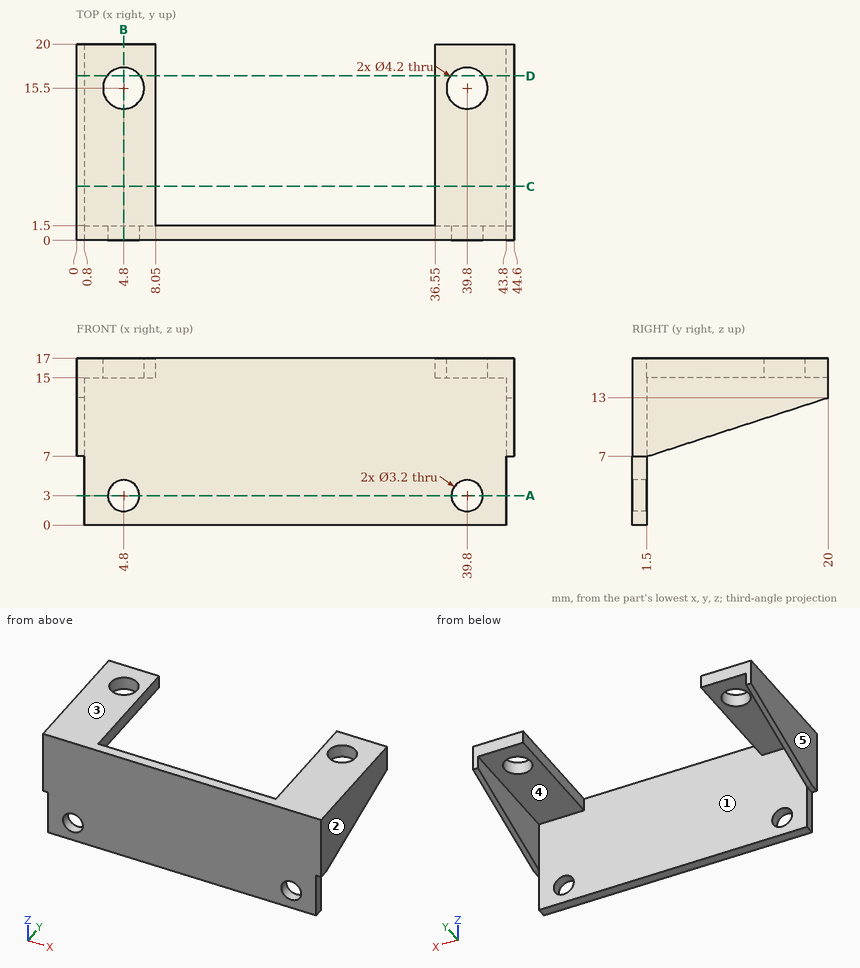
Input: dimensioned drawing with shaded views. Units: mm. Origin: part minimum x, y, z. A direction names the side the tool comes from. Coordinates: 2 decimals unless noted, no trailing zeros. Loops run counter-clockwise (first coordinate to the right, second up) from the corner with the lowest first, then second, coordinate; pieces in that order, holes last. Notation, with made-up numbers: M 83,-21.5 L 117,-21.5 A9 ccw 117,-13.5 Z; hole C 40.25,42 d8. An arc over 180 degrees is marked long. Use a Markdown table: item, result. Add a question column.
Q1. Section query D-D, the plane y = 16.75. Return loops of the section in (x, z).
Q2. Section query B-B, the plane x = 4.8. Return loops of the section in (y, z), and give its area (3 significant figures).
Q3. Material intervals for L1, parallel to X at y = 1, z = 3; L2, parallel to Y at x = 39.8, z = 16.1; L3, parallel to X at y = 3, z = 9.25, sorted ascending.
Q4. Draft query along X for the marked faces 1, 2 and 3. Return one class per face: pulls with the +X half, pulls with the -X half, needs draft (parallel to the pull), parting line crosses it, or undercut.
Q5. Access query for the marked faces 4 and 5. Directions: +Z, -Z, +X, -X, +Y, -Y. A direction counts if a zero-diameter tool reaches every point of the face in a straight line with its end or side. Return the directions, or none.
Q6. First-contact query: pin 1 (1.5 mm diameter, centred on x = 25, y = 3, fed in from +Z); pin 2 (0.8 mm diameter, centred on y = 1, z = 3, fed in from -X); pin 3 (12 mm diameter, centred on x = 13.5, y = 8, fed in from -Z); pin 4 (8 mm diameter, centred on x = 11.5, z = 4.5, fed in from +Y). Flat tips, straight axial feed; report the tip coordinate or a pass-through.
Q7. Section query C-C, the plane y = 5.5. Return loops of the section in (x, z).
Q8. Section query A-A, the plane z = 3. Return loops of the section in (x, y), and give its area (3 significant figures).
Result:
| question | item | result |
|---|---|---|
| 1 | outline | M 0,11.95 L 0.8,11.95 L 0.8,15 L 3.11,15 L 3.11,17 L 0,17 Z; M 6.49,15 L 8.05,15 L 8.05,17 L 6.49,17 Z; M 36.55,15 L 38.11,15 L 38.11,17 L 36.55,17 Z; M 41.49,15 L 43.8,15 L 43.8,11.95 L 44.6,11.95 L 44.6,17 L 41.49,17 Z |
| 2 | outline | M 0,0 L 1.5,0 L 1.5,1.4 L 0,1.4 Z; M 0,4.6 L 1.5,4.6 L 1.5,15 L 13.4,15 L 13.4,17 L 0,17 Z; M 17.6,15 L 20,15 L 20,17 L 17.6,17 Z |
| 2 | area | 49.3 mm2 |
| 3 | L1 | x = 0.8 to 3.2, 6.4 to 38.2, 41.4 to 43.8 |
| 3 | L2 | y = 0 to 13.4, 17.6 to 20 |
| 3 | L3 | x = 0 to 0.8, 43.8 to 44.6 |
| 4 | face 1 | undercut |
| 4 | face 2 | pulls with the +X half |
| 4 | face 3 | needs draft |
| 5 | face 4 | -Z, +Y |
| 5 | face 5 | +Z, -Z, -X, +Y, -Y |
| 6 | pin 1 | passes through |
| 6 | pin 2 | stops at x = 0.8 |
| 6 | pin 3 | stops at z = 15 |
| 6 | pin 4 | stops at y = 1.5 |
| 7 | outline | M 0,8.3 L 0.8,8.3 L 0.8,15 L 8.05,15 L 8.05,17 L 0,17 Z; M 36.55,15 L 43.8,15 L 43.8,8.3 L 44.6,8.3 L 44.6,17 L 36.55,17 Z |
| 8 | outline | M 0.8,0 L 3.2,0 L 3.2,1.5 L 0.8,1.5 Z; M 6.4,0 L 38.2,0 L 38.2,1.5 L 6.4,1.5 Z; M 41.4,0 L 43.8,0 L 43.8,1.5 L 41.4,1.5 Z |
| 8 | area | 54.9 mm2 |
